from build123d import *

# Parameters (mm, degrees)
EXTRUDE_1_DEPTH     = 16
SKETCH_2_W          = 11.421069603
SKETCH_2_H          = 55.615643281
CUT_EXTRUDE_1_DEPTH = 16
SKETCH_3_R          = 1.6
CUT_EXTRUDE_2_DEPTH = 16


with BuildPart() as part:
    # 草图1 → 凸台-拉伸1 (new body)
    with BuildSketch(Plane.XY):
        Polygon((0, 3), (0, 0), (5, 0), (15, 0), (15, 3), (5, 3), (5, 63), (0, 63), align=None)
    extrude(amount=EXTRUDE_1_DEPTH)

    # 草图2 → 切除-拉伸1 (cut)
    with BuildSketch(Plane(origin=(5, 0, 0), x_dir=(0, 0, -1), z_dir=(1, 0, 0))):
        with Locations((-8.070938321, 32.244852366)):
            Rectangle(SKETCH_2_W, SKETCH_2_H)
    extrude(amount=-CUT_EXTRUDE_1_DEPTH, mode=Mode.SUBTRACT)

    # 草图3 → 切除-拉伸2 (cut)
    with BuildSketch(Plane(origin=(0, 3, 0), x_dir=(1, 0, 0), z_dir=(0, 1, 0))):
        with Locations(Location((9.503642987, -8.058930676, 0), (0, 0, 270))):
            Circle(SKETCH_3_R)
    extrude(amount=-CUT_EXTRUDE_2_DEPTH, mode=Mode.SUBTRACT)


solid = part.part
Check sheet for the modelled part. Datum: model origin and axes. Units: mm. A direction names the side the tool comes from. Round coordinates to 2 decimals unless told otherwise and drop trailing zeros. Loops run counter-clockwise (first coordinate to the right, second up) from the corner with the lowest first, then second, coordinate; pieces in that order, holes last.
1. Sectioned sample at D-D on x = 6.75. Record the boundary of the cut face in (y, z).
2. Scan lines: probe 1 along Z at (x, y) = (4.75, 29.5); probe 2 along Y at (x, z) = (3.25, 13); probe 3 along Y at (x, z) = (7.5, 2.75). Record each from-to range of solid material in increasing order.
3. Gauge pin test, flat ends, axial feed: pin 1 Ø5 at (x, z) = (9, 4) entering from +Y; pin 2 Ø4 at (x, y) = (7.5, 43.5) entering from -Z; pin 3 Ø8 at (y, z) = (46.5, 5.5) entering from +X. Record the tip position at first contact, or that the pin passes through.
4. Mould release check, pull along Z, two halves, no side actions. Record for faces 1 (the flat face through (2, 29, 16)), 2 (the flat face through (3, 60.053, 8)), 3 (the flat face through (7, 0, 8)): released by +Z, released by -Z, zero draft, split by the parting line, or undercut.
5. Sectioned sample at A-A on y = 26. Record the boundary of the cut face in (x, z), and give its area (3 significant figures).
6. Set-up check for faces 4 (the flat face through (15, 1, 8)), 5 (the flat face through (3, 32, 13.781)), 6 (the flat face through (10, 3, 10)): record each of +Z, -Z, +X, -X, +Y, -Y from which the full face is reachable in a straight line by a thin tool's end or side.
7. Sectioned sample at C-C on z = 1.5. Record the boundary of the cut face in (x, y).
8. Sectioned sample at B-B on x = 3. Record the boundary of the cut face in (y, z), and give its area (3 significant figures).
Recorded:
1. outline: (0, 0) - (3, 0) - (3, 16) - (0, 16) - close
2. probe 1: z = 0 to 2.36, 13.78 to 16
2. probe 2: y = 0 to 4.44, 60.05 to 63
2. probe 3: y = 0 to 3
3. pin 1: stops at y = 3
3. pin 2: passes through
3. pin 3: stops at x = 5
4. face 1: released by +Z
4. face 2: undercut
4. face 3: zero draft
5. outline: (0, 0) - (5, 0) - (5, 2.36) - (0, 2.36) - close; (0, 13.78) - (5, 13.78) - (5, 16) - (0, 16) - close
5. area: 22.9 mm2
6. face 4: +Z, -Z, +X, +Y, -Y
6. face 5: +X, -X
6. face 6: +Z, -Z, +X, +Y
7. outline: (0, 0) - (15, 0) - (15, 3) - (5, 3) - (5, 63) - (0, 63) - close
8. outline: (0, 0) - (63, 0) - (63, 16) - (0, 16) - close; hole (4.44, 2.36) - (60.05, 2.36) - (60.05, 13.78) - (4.44, 13.78) - close
8. area: 373 mm2
